```python
from build123d import *

# Parameters (mm, degrees)
SKETCH_1_W          = 10
SKETCH_1_H          = 15
SKETCH_1_W_2        = 8
SKETCH_1_H_2        = 12
EXTRUDE_1_DEPTH     = 40
SKETCH_2_R          = 1.6
CUT_EXTRUDE_1_DEPTH = 44.011626335
SKETCH_3_R          = 1.6
CUT_EXTRUDE_2_DEPTH = 42.907636536


with BuildPart() as part:
    # ｽｹｯﾁ1 → ﾎﾞｽ - 押し出し1 (new body)
    with BuildSketch(Plane.XY):
        Rectangle(SKETCH_1_W, SKETCH_1_H)
        Rectangle(SKETCH_1_W_2, SKETCH_1_H_2, mode=Mode.SUBTRACT)
    extrude(amount=EXTRUDE_1_DEPTH)

    # ｽｹｯﾁ2 → ｶｯﾄ - 押し出し1 (cut, through all)
    with BuildSketch(Plane(origin=(0, 7.5, 0), x_dir=(1, 0, 0), z_dir=(0, 1, 0))):
        with Locations(Location((0, -20, 0), (0, 0, 270))):
            Circle(SKETCH_2_R)
    extrude(amount=-CUT_EXTRUDE_1_DEPTH, mode=Mode.SUBTRACT)

    # ｽｹｯﾁ3 → ｶｯﾄ - 押し出し2 (cut, through all)
    with BuildSketch(Plane(origin=(5, 0, 0), x_dir=(0, 0, -1), z_dir=(1, 0, 0))):
        with Locations(Location((-35, -2.5, 0), (0, 0, 90))):
            Circle(SKETCH_3_R)
        with Locations(Location((-5, -2.5, 0), (0, 0, 90))):
            Circle(SKETCH_3_R)
    extrude(amount=-CUT_EXTRUDE_2_DEPTH, mode=Mode.SUBTRACT)


solid = part.part
```
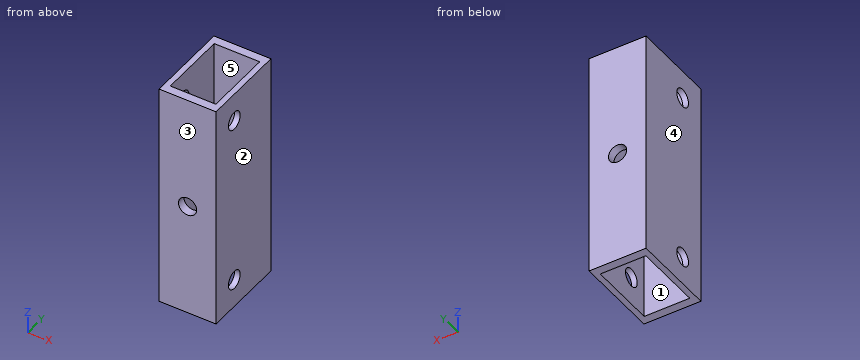
Source: CAD feature listing. Evaluate the final solid. Frame: model axes, mm. Face numbers are marked on the shaded views. A direction names the side the tool comes from. Round coordinates to 2 decimals unless told otherwise and drop trailing zeros. Order: outer loops, then holes, each group sorted by start corner. A loop starts at its lowest first (then second) coordinate and runs counter-clockwise, first axis right, second up. Notation, with made-up numbers: (28.5, 62.25) -> (36.5, 62.25) arc R10 cw to (36.5, 77.25) -> close; hole circle Ø6 at (67.25, -17.5). An arc over 180 degrees is marked (long way). One line per item, written item: value. Start each with the question number.
Q1. Pin query (flat end, axial travel): pin 1 (3.5 mm diameter, centred on y = -2.5, z = 35, fed in from +X). Return the tip coordinate at first contact, or that it passes through.
Q2. Section query B-B (z = 5). Return the cut outline in (x, y), plus the area to 3 significant figures.
Q3. Material intervals for probe 1 along Z at (x, y) = (4.65, -2.5); probe 2 along Y at (x, z) = (-0.5, 4); probe 3 along X at (y, z) = (-6.35, 20), sorted ascending.
Q4. Draft query along X for the marked faces 3, 4 and 5. Return one class per face: pulls with the +X half, pulls with the -X half, needs draft (parallel to the pull), parting line crosses it, or undercut.
Q5. Section query D-D (y = -2.5). Return the cut outline in (x, z).
Q6. Section query A-A (x = -3). Return the cut outline in (y, z).
Q7. Access query for the marked faces 1 and 2. Directions: +Z, -Z, +X, -X, +Y, -Y. A direction counts if a zero-diameter tool reaches every point of the face in a straight line with its end or side. Return the directions, or none.
Q8. Section query C-C (y = -0.5). Return the cut outline in (x, z).
Findings below:
1. pin 1: x = 5
2. outline: (-5, -7.5) -> (5, -7.5) -> (5, -4.1) -> (4, -4.1) -> (4, -6) -> (-4, -6) -> (-4, -4.1) -> (-5, -4.1) -> close; (-5, -0.9) -> (-4, -0.9) -> (-4, 6) -> (4, 6) -> (4, -0.9) -> (5, -0.9) -> (5, 7.5) -> (-5, 7.5) -> close
2. area: 47.6 mm²
3. probe 1: 0 to 3.4, 6.6 to 33.4, 36.6 to 40
3. probe 2: -7.5 to -6, 6 to 7.5
3. probe 3: -5 to -1.6, 1.6 to 5
4. face 3: needs draft
4. face 4: pulls with the -X half
4. face 5: undercut
5. outline: (-5, 0) -> (-4, 0) -> (-4, 3.4) -> (-5, 3.4) -> close; (-5, 6.6) -> (-4, 6.6) -> (-4, 33.4) -> (-5, 33.4) -> close; (-5, 36.6) -> (-4, 36.6) -> (-4, 40) -> (-5, 40) -> close; (4, 0) -> (5, 0) -> (5, 3.4) -> (4, 3.4) -> close; (4, 6.6) -> (5, 6.6) -> (5, 33.4) -> (4, 33.4) -> close; (4, 36.6) -> (5, 36.6) -> (5, 40) -> (4, 40) -> close
6. outline: (-7.5, 0) -> (-6, 0) -> (-6, 40) -> (-7.5, 40) -> close; (6, 0) -> (7.5, 0) -> (7.5, 40) -> (6, 40) -> close
7. face 1: +Z, -Z
7. face 2: +Z, -Z, +X, +Y, -Y
8. outline: (-5, 0) -> (-4, 0) -> (-4, 40) -> (-5, 40) -> close; (4, 0) -> (5, 0) -> (5, 40) -> (4, 40) -> close
